Design review of the part built by this model. Coordinates are the model's own, in mm. Give positions to 0.01 mm unless a question says otherwise; leave off trailing zeros. Order: outer loops, then holes, each group sorted by start corner. A loop starts at its lowest first (then second) coordinate and runs counter-clockwise, first axis right, second up. Notation, with made-up numbers: (60.25, -20.75) -> (66.25, -20.75) arc R16 cw to (66.25, -10.75) -> close; hole circle Ø3 at (-31, 43). An arc over 180 degrees is marked (long way). Return JSON: item names as keys, results as strings.
Autodesk Inventor part; units mm, degrees
ref_plane "YZ Plane" through (0, 0, 0) normal (1, 0, 0) x (0, 1, 0)
ref_plane "XZ Plane" through (0, 0, 0) normal (0, 1, 0) x (-1, 0, 0)
ref_plane "XY Plane" through (0, 0, 0) normal (0, 0, 1) x (1, 0, 0)
sketch "Эскиз1" plane through (0, 0, 0) normal (0, 0, 1) x (1, 0, 0)
  line L0 (0, 0) -> (29.6206, 0)
  line L1 (0, 0) -> (0, 38)
  line L2 (2, 40) -> (3.25, 40)
  arc A0 (2, 40) -> (0, 38) centre (2, 38) ccw
  line L3 (3.25, 45) -> (2, 45)
  arc A1 (2, 45) -> (-5, 38) centre (2, 38) ccw
  line L4 (-5, 38) -> (-5, 0)
  line L5 (-5, 0) -> (0, 0)
  line L6 (3.25, 45) -> (3.25, 40)
  dimension "d0" = 80
  dimension "d1" = 2
  dimension "d2" = 90
  dimension "d5" = 8.25
revolve "Вращение1" add sketch "Эскиз1" angle 360 about axis through (0, 0, 0) along (1, 0, 0)
properties part number "Регулировка-тихая"
Item 1: Wall thickness on L1, parallel to Z at x = 2.9, y = 0; L2, parallel to X at y = -35, z = 3; L3, parallel to Z at x = 0.75, y = -4: over which ranges is each line inside the solid? List them lowest first. Write a range as [from, to].
Result set:
{"L1": "z = [-45, -40], [40, 45]", "L2": "x = [-5, 0]", "L3": "z = [-44.71, -39.36], [39.36, 44.71]"}
Item 2: Add section A-A (y = 0). Give the boundary of the cut face in (x, z), plus the area to 3 significant figures.
Result set:
{"outline": "(-5, -38) arc R7 ccw to (2, -45) -> (3.25, -45) -> (3.25, -40) -> (2, -40) arc R2 cw to (0, -38) -> (0, 38) arc R2 cw to (2, 40) -> (3.25, 40) -> (3.25, 45) -> (2, 45) arc R7 ccw to (-5, 38) -> close", "area": "463 mm^2"}
Item 3: Mouldability with a two-part tool opening along Z and no side actions: class faces 1 (the face through (3.25, -30.2, -26.5)), 2 (the face through (0, -1, 1)), 3 (the face through (2.63, -8.67, -39.05)), 4 (the face through (2.616, 20.765, 39.923)) as released by +Z, released by -Z, zero draft, split by the parting line, or undercut.
Result set:
{"face 1": "zero draft", "face 2": "undercut", "face 3": "undercut", "face 4": "split by the parting line"}
Item 4: For pin 1 (1 mm diameter, centred on x = -3, y = 16, fed in from +Z); pin 2 (1.5 mm diameter, centred on x = 2, z = -32.5, fed in from -Y); pin 3 (2 mm diameter, centred on y = -33.5, z = -6, fed in from +X), all flat-tipped, find the tip position at first contact; note any pin that passes through.
Result set:
{"pin 1": "stops at z = 40.34", "pin 2": "stops at y = -31.89", "pin 3": "stops at x = 0"}
Item 5: Add section B-B (x = -3). Give the boundary of the cut face in (y, z), plus the area to 3 significant figures.
Result set:
{"outline": "circle Ø85.8 at (0, 0)", "area": "5,780 mm^2"}
